```python
from build123d import *

# Parameters (mm, degrees)
SKETCH1_W           = 240
SKETCH1_H           = 240
BOSS_EXTRUDE1_DEPTH = 6
SKETCH2_R           = 1.75
CUT_EXTRUDE1_DEPTH  = 170.811660377
SKETCH4_R           = 2.75
CUT_EXTRUDE2_DEPTH  = 170.811660377
SKETCH5_W           = 190
SKETCH5_H           = 120
SKETCH5_H_2         = 30
CUT_EXTRUDE3_DEPTH  = 170.811660377
SKETCH6_R           = 11.5
CUT_EXTRUDE4_DEPTH  = 170.811660377
SKETCH9_R           = 2.75
CUT_EXTRUDE7_DEPTH  = 10
SKETCH10_R          = 1.75
CUT_EXTRUDE8_DEPTH  = 10
SKETCH11_R          = 1.75
CUT_EXTRUDE9_DEPTH  = 10
FILLET1_R           = 10


with BuildPart() as part:
    # Sketch1 → Boss-Extrude1 (new body)
    with BuildSketch(Plane(origin=(0, 0, 0), x_dir=(1, 0, 0), z_dir=(0, 1, 0))):
        Rectangle(SKETCH1_W, SKETCH1_H)
    extrude(amount=BOSS_EXTRUDE1_DEPTH)

    # Sketch2 → Cut-Extrude1 (cut, through all)
    with BuildSketch(Plane(origin=(0, 6, 0), x_dir=(1, 0, 0), z_dir=(0, 1, 0))):
        with Locations(Location((105.5, 33, 0), (0, 0, 270))):
            Circle(SKETCH2_R)
        with Locations(Location((105.5, 13, 0), (0, 0, 270))):
            Circle(SKETCH2_R)
        with Locations(Location((105.5, -7, 0), (0, 0, 270))):
            Circle(SKETCH2_R)
        with Locations(Location((105.5, -27, 0), (0, 0, 270))):
            Circle(SKETCH2_R)
        with Locations(Location((105.5, -47, 0), (0, 0, 270))):
            Circle(SKETCH2_R)
        with Locations(Location((105.5, -67, 0), (0, 0, 270))):
            Circle(SKETCH2_R)
        with Locations(Location((105.5, -87, 0), (0, 0, 270))):
            Circle(SKETCH2_R)
        with BuildLine():
            Line((71.5, 105.75), (71.5, 107.5))
            Line((71.5, 107.5), (73.25, 107.5))
            ThreePointArc((73.25, 107.5), (70.262563133, 108.737436867), (71.5, 105.75))
        make_face()
        with BuildLine():
            Line((73.25, 107.5), (71.5, 107.5))
            Line((71.5, 107.5), (71.5, 105.75))
            ThreePointArc((71.5, 105.75), (72.737436867, 106.262563133), (73.25, 107.5))
        make_face()
        with BuildLine():
            ThreePointArc((104.25, 107.5), (102.5, 109.25), (100.75, 107.5))
            Line((100.75, 107.5), (102.5, 107.5))
            Line((102.5, 107.5), (102.5, 105.75))
            ThreePointArc((102.5, 105.75), (103.737436867, 106.262563133), (104.25, 107.5))
        make_face()
        with BuildLine():
            Line((102.5, 107.5), (100.75, 107.5))
            ThreePointArc((100.75, 107.5), (101.262563133, 106.262563133), (102.5, 105.75))
            Line((102.5, 105.75), (102.5, 107.5))
        make_face()
        with BuildLine():
            ThreePointArc((104.25, 76.5), (103.737436867, 77.737436867), (102.5, 78.25))
            Line((102.5, 78.25), (102.5, 76.5))
            Line((102.5, 76.5), (100.75, 76.5))
            ThreePointArc((100.75, 76.5), (102.5, 74.75), (104.25, 76.5))
        make_face()
        with BuildLine():
            Line((102.5, 76.5), (102.5, 78.25))
            ThreePointArc((102.5, 78.25), (101.262563133, 77.737436867), (100.75, 76.5))
            Line((100.75, 76.5), (102.5, 76.5))
        make_face()
        with BuildLine():
            ThreePointArc((73.25, 76.5), (72.737436867, 77.737436867), (71.5, 78.25))
            Line((71.5, 78.25), (71.5, 76.5))
            Line((71.5, 76.5), (73.25, 76.5))
        make_face()
        with BuildLine():
            Line((71.5, 76.5), (71.5, 78.25))
            ThreePointArc((71.5, 78.25), (70.262563133, 75.262563133), (73.25, 76.5))
            Line((73.25, 76.5), (71.5, 76.5))
        make_face()
        with Locations(Location((105.5, 53, 0), (0, 0, 270))):
            Circle(SKETCH2_R)
    cut_extrude1 = extrude(amount=-CUT_EXTRUDE1_DEPTH, mode=Mode.SUBTRACT)

    # Mirror1: Cut-Extrude1 across plane
    add(cut_extrude1.mirror(Plane(origin=(0, 0, 0), x_dir=(0, 0, 1), z_dir=(1, 0, 0))), mode=Mode.SUBTRACT)

    # Sketch4 → Cut-Extrude2 (cut, through all)
    with BuildSketch(Plane(origin=(0, 6, 0), x_dir=(1, 0, 0), z_dir=(0, 1, 0))):
        with Locations(Location((-87, -105, 0), (0, 0, 270))):
            Circle(SKETCH4_R)
    cut_extrude2 = extrude(amount=-CUT_EXTRUDE2_DEPTH, mode=Mode.SUBTRACT)

    # Mirror2: Cut-Extrude2 across plane
    add(cut_extrude2.mirror(Plane(origin=(0, 0, 0), x_dir=(0, 0, 1), z_dir=(1, 0, 0))), mode=Mode.SUBTRACT)

    # Sketch5 → Cut-Extrude3 (cut, through all)
    with BuildSketch(Plane(origin=(0, 6, 0), x_dir=(1, 0, 0), z_dir=(0, 1, 0))):
        Rectangle(SKETCH5_W, SKETCH5_H)
        with Locations((0, -75)):
            Rectangle(SKETCH5_W, SKETCH5_H_2)
    extrude(amount=-CUT_EXTRUDE3_DEPTH, mode=Mode.SUBTRACT)

    # Sketch6 → Cut-Extrude4 (cut, through all)
    with BuildSketch(Plane(origin=(0, 6, 0), x_dir=(1, 0, 0), z_dir=(0, 1, 0))):
        with Locations(Location((-87, 91.6, 0), (0, 0, 270))):
            Circle(SKETCH6_R)
    cut_extrude4 = extrude(amount=-CUT_EXTRUDE4_DEPTH, mode=Mode.SUBTRACT)

    # Mirror3: Cut-Extrude4 across plane
    add(cut_extrude4.mirror(Plane(origin=(0, 0, 0), x_dir=(0, 0, 1), z_dir=(1, 0, 0))), mode=Mode.SUBTRACT)

    # Sketch9 → Cut-Extrude7 (cut)
    with BuildSketch(Plane(origin=(0, 6, 0), x_dir=(1, 0, 0), z_dir=(0, 1, 0))):
        with Locations(Location((-109, -113, 0), (0, 0, 270))):
            Circle(SKETCH9_R)
        with Locations(Location((-65, -113, 0), (0, 0, 90))):
            Circle(SKETCH9_R)
        with Locations(Location((65, -113, 0), (0, 0, 270))):
            Circle(SKETCH9_R)
        with Locations(Location((109, -113, 0), (0, 0, 90))):
            Circle(SKETCH9_R)
    extrude(amount=-CUT_EXTRUDE7_DEPTH, mode=Mode.SUBTRACT)

    # Sketch10 → Cut-Extrude8 (cut)
    with BuildSketch(Plane(origin=(0, 6, 0), x_dir=(1, 0, 0), z_dir=(0, 1, 0))):
        with Locations(Location((-105.5, 65, 0), (0, 0, 270))):
            Circle(SKETCH10_R)
    cut_extrude8 = extrude(amount=-CUT_EXTRUDE8_DEPTH, mode=Mode.SUBTRACT)

    # Mirror4: Cut-Extrude8 across plane
    add(cut_extrude8.mirror(Plane(origin=(0, 0, 0), x_dir=(0, 0, 1), z_dir=(1, 0, 0))), mode=Mode.SUBTRACT)

    # Sketch11 → Cut-Extrude9 (cut)
    with BuildSketch(Plane(origin=(0, 6, 0), x_dir=(1, 0, 0), z_dir=(0, 1, 0))):
        with Locations(Location((-105.5, -98.5, 0), (0, 0, 270))):
            Circle(SKETCH11_R)
    cut_extrude9 = extrude(amount=-CUT_EXTRUDE9_DEPTH, mode=Mode.SUBTRACT)

    # Mirror6: Cut-Extrude9 across plane
    add(cut_extrude9.mirror(Plane(origin=(0, 0, 0), x_dir=(0, 0, 1), z_dir=(1, 0, 0))), mode=Mode.SUBTRACT)

    # Fillet1
    fillet1_edges = [part.edges().sort_by_distance(p)[0] for p in [
        (-95, 3, 90),
        (-95, 3, -60),
        (95, 3, -60),
        (95, 3, 90),
        (120, 3, 120),
        (-120, 3, 120),
        (-120, 3, -120),
        (120, 3, -120),
    ]]
    fillet(fillet1_edges, radius=FILLET1_R)


solid = part.part
```
CAD build for the part. Positions are in the model's coordinates, mm. A direction names the side the tool comes from. Coordinates: 2 decimals unless noted, no trailing zeros. Order: outer loops, then holes, each group sorted by start corner. A loop starts at its lowest first (then second) coordinate and runs counter-clockwise, first axis right, second up. Notation, with made-up numbers: (43.5, 13) - (60.5, 13) arc R8 cw to (60.5, 23) - close; hole circle Ø9 at (-32, 27). An arc over 180 degrees is marked (long way). Use a Markdown table: item, result. Add a question column.
(1) Saw through at B-B (x = 8). Give the cut face in (y, z).
(2) Pull direction Z, two halves, no side cores. Call faces 3 (the face through (-117.15, 3.04, 116.99)), 4 (the face through (-2, 6, -82)), 5 (the face through (111.685, 3.042, 113.596)), 6 (the face through (-2, 3, -120)): +Z half, -Z half, draft (parallel to the pull), parting line (faces both ways), or undercut.
(3) Saw through at A-A (z = 37). Give the cut face in (x, y), then the cut area to 3 significant figures.
(4) Flat gauge pin, fed straight in: pin 1 (3 mm diameter, centred on x = 105.5, z = 7, fed in from -Y). Where does the tip first touch, or does it go through?
(5) Which spindle directions (+Z, -Z, +X, -X, +Y, -Y) get a long thin tool onto all of the face, cutting with end or side? Do faces 1 (the face through (116.99, 3.04, 117.15)), 2 (the face through (-1, 3, 90)). Say none if no direction does.
(6) Saw through at C-C (y = 3.5). Count the separate pieces of the cut face and the enclosed holes in it, then the cut area to 3 significant figures.
(7) Drill centre lines: line 1 along X through (y, z) = (3.85, -107.5); line 2 along X through (y, z) = (4.1, 16); line 3 along Z through (x, y) = (-51, 4.4). Where is each one in solid material? Low to high. Write a range as [from, to].
Solved:
| question | item | result |
|---|---|---|
| 1 | outline | (0, -120) - (6, -120) - (6, -60) - (0, -60) - close; (0, 90) - (6, 90) - (6, 120) - (0, 120) - close |
| 2 | face 3 | +Z half |
| 2 | face 4 | draft |
| 2 | face 5 | undercut |
| 2 | face 6 | -Z half |
| 3 | outline | (-120, 0) - (-95, 0) - (-95, 6) - (-120, 6) - close; (95, 0) - (120, 0) - (120, 6) - (95, 6) - close |
| 3 | area | 300 mm² |
| 4 | pin 1 | passes through |
| 5 | face 1 | +Z, +X, +Y, -Y |
| 5 | face 2 | +Y, -Y |
| 6 | separate pieces | 1 |
| 6 | enclosed holes | 37 |
| 6 | area | 27,900 mm² |
| 7 | line 1 | x = [-120, -104.25], [-100.75, -73.25], [-69.75, 69.75], [73.25, 100.75], [104.25, 120] |
| 7 | line 2 | x = [-120, -95], [95, 120] |
| 7 | line 3 | z = [-120, -60], [90, 120] |
